Autodesk Inventor part; units mm, degrees
ref_plane "YZ Plane" through (0, 0, 0) normal (1, 0, 0) x (0, 1, 0)
ref_plane "XZ Plane" through (0, 0, 0) normal (0, 1, 0) x (-1, 0, 0)
ref_plane "XY Plane" through (0, 0, 0) normal (0, 0, 1) x (1, 0, 0)
sketch "Sketch1" plane through (0, 0, 0) normal (1, 0, 0) x (0, 1, 0)
  line L0 (0, 0) -> (0, 4.3483) construction
  line L1 (2.5, 0) -> (2.5, 5)
  line L2 (2.5, 5) -> (3.5, 5)
  line L3 (3.5, 5) -> (3.5, 4.75)
  line L4 (3.5, 4.75) -> (7, 4.75)
  line L5 (7, 4.75) -> (7, 5)
  line L6 (7, 5) -> (8, 5)
  line L7 (8, 5) -> (8, 0)
  line L8 (8, 0) -> (7, 0)
  line L9 (7, 0) -> (7, 0.25)
  line L10 (7, 0.25) -> (3.5, 0.25)
  line L11 (3.5, 0.25) -> (3.5, 0)
  line L12 (3.5, 0) -> (2.5, 0)
  line L13 (0, 0) -> (12.4665, 0) construction
  dimension "d0" = 5
  dimension "d1" = 16
  dimension "d2" = 1
  dimension "d3" = 1
  dimension "d4" = 0.25
  dimension "d5" = 0.25
  dimension "d6" = 5
revolve "Revolution1" add sketch "Sketch1" angle 360 about axis through (0, 0, 0) along (0, 0, 1)
properties part number "Ball Bearing 625 2RS 5x16x5"
Verification items for the finished model (mm, model axes). A direction names the side the tool comes from. Coordinates: 2 decimals unless noted, no trailing zeros. Order: outer loops, then holes, each group sorted by start corner. A loop starts at its lowest first (then second) coordinate and runs counter-clockwise, first axis right, second up. Notation, with made-up numbers: (-4.5, 3.25) -> (18.5, 3.25) arc R25 cw to (18.5, 34.25) -> close; hole circle Ø11 at (19, 46). An arc over 180 degrees is marked (long way). Put each result on its own line as item: value. Start each with the question number.
1) Cross-section at C-C (z = 2.4). Enter the section's corners in (x, y), plus the area to 3 significant figures.
2) Tool access check on faces 4 (the flat face through (3, 3, 4.75)), 5 (the flat face through (6, 4, 5)), 6 (the flat face through (3, 3, 0.25)). Record the directions out of +Z, -Z, +X, -X, +Y, -Y that give a thin tool (end or side, any length) a straight path to the whole face; none if there is none.
3) Release check for a two-part mould opening along X. For faces 1 (the flat face through (2, 2, 5)), 2 (the cylindrical face through (2.44, -0.54, 2.54)), 3 (the cylindrical face through (-7.81, -1.73, 2.46)) record: pulls with the +X half, pulls with the -X half, needs draft (parallel to the pull), parting line crosses it, or undercut.
4) Cross-section at A-A (x = 0). Enter the section's corners in (y, z).
5) Material ranges on L1, parallel to X at y = 0, z = 0.1; L2, parallel to X at y = 0, z = 2.3, recorded low to high.
6) Cross-section at D-D (y = 6.5). Enter the section's corners in (x, z), plus the area to 3 significant figures.
Geometry check:
1. outline: circle Ø16 at (0, 0); hole circle Ø5 at (0, 0)
1. area: 181 mm^2
2. face 4: +Z
2. face 5: +Z, +X, -X, +Y, -Y
2. face 6: -Z
3. face 1: needs draft
3. face 2: undercut
3. face 3: parting line crosses it
4. outline: (-8, 0) -> (-7, 0) -> (-7, 0.25) -> (-3.5, 0.25) -> (-3.5, 0) -> (-2.5, 0) -> (-2.5, 5) -> (-3.5, 5) -> (-3.5, 4.75) -> (-7, 4.75) -> (-7, 5) -> (-8, 5) -> close; (2.5, 0) -> (3.5, 0) -> (3.5, 0.25) -> (7, 0.25) -> (7, 0) -> (8, 0) -> (8, 5) -> (7, 5) -> (7, 4.75) -> (3.5, 4.75) -> (3.5, 5) -> (2.5, 5) -> close
5. L1: x = -8 to -7, -3.5 to -2.5, 2.5 to 3.5, 7 to 8
5. L2: x = -8 to -2.5, 2.5 to 8
6. outline: (-4.66, 0) -> (-2.6, 0) -> (-2.6, 0.25) -> (2.6, 0.25) -> (2.6, 0) -> (4.66, 0) -> (4.66, 5) -> (2.6, 5) -> (2.6, 4.75) -> (-2.6, 4.75) -> (-2.6, 5) -> (-4.66, 5) -> close
6. area: 44.0 mm^2
